from build123d import *

# Parameters (mm, degrees)
SKETCH022_AS_DRAWN_R                      = 2.7
EXTRUDE013_DEPTH                          = 25.4
EXTRUDE013_ONTO_SKETCH022_PLACEMENT_ANGLE = 8
SKETCH018_AS_DRAWN_R                      = 1.2
EXTRUDE009_DEPTH                          = 7.8
EXTRUDE009_ONTO_SKETCH018_PLACEMENT_ANGLE = 8
EXTRUDE012_DEPTH                          = 6.35
EXTRUDE012_ONTO_SKETCH021_PLACEMENT_ANGLE = 8


with BuildPart() as top_led_holes:
    # Sketch022 as drawn → Extrude013 (new, symmetric)
    with BuildSketch(Plane.XY):
        with Locations((116.082414, 49.440535)):
            Circle(SKETCH022_AS_DRAWN_R)
        with Locations((97.448702, 45.479818)):
            Circle(SKETCH022_AS_DRAWN_R)
        with Locations((78.81499, 41.5191)):
            Circle(SKETCH022_AS_DRAWN_R)
    extrude(amount=EXTRUDE013_DEPTH, both=True)


with BuildPart() as top_led_holes_1:
    # Extrude013 onto Sketch022 placement: moved
    add(top_led_holes.part.moved(Location((42.3672, 0, 47.625))).rotate(Axis((42.3672, 0, 47.625), (0, 1, 0)), EXTRUDE013_ONTO_SKETCH022_PLACEMENT_ANGLE))


with BuildPart() as screw_hole_cuts:
    # Sketch018 as drawn → Extrude009 (new)
    with BuildSketch(Plane.XY):
        with Locations((-31.998318, 84.649891)):
            Circle(SKETCH018_AS_DRAWN_R)
        with Locations((-31.998318, -89.695043)):
            Circle(SKETCH018_AS_DRAWN_R)
        with Locations((156.654735, -49.595599)):
            Circle(SKETCH018_AS_DRAWN_R)
        with Locations((156.654735, 84.649891)):
            Circle(SKETCH018_AS_DRAWN_R)
    extrude(amount=EXTRUDE009_DEPTH)


with BuildPart() as screw_hole_cuts_1:
    # Extrude009 onto Sketch018 placement: moved
    add(screw_hole_cuts.part.moved(Location((39.98734, 0, 30.691416))).rotate(Axis((39.98734, 0, 30.691416), (0, 1, 0)), EXTRUDE009_ONTO_SKETCH018_PLACEMENT_ANGLE))


with BuildPart() as cut006:
    # Sketch021 as drawn → Extrude012 (new)
    with BuildSketch(Plane.XY):
        Polygon((-39.826537, 91.531891), (-39.826537, -98.44048), (161.021837, -55.74884), (163.536735, -52.643218), (163.536735, 88.356895), (160.361736, 91.531891), align=None)
    extrude(amount=EXTRUDE012_DEPTH)


with BuildPart() as cut006_1:
    # Extrude012 onto Sketch021 placement: moved
    add(cut006.part.moved(Location((40.182182, 0, 32.077791))).rotate(Axis((40.182182, 0, 32.077791), (0, 1, 0)), EXTRUDE012_ONTO_SKETCH021_PLACEMENT_ANGLE))

    # Cut004: cut Screw Hole Cuts
    add(screw_hole_cuts_1.part, mode=Mode.SUBTRACT)

    # Cut006: cut Top LED Holes
    add(top_led_holes_1.part, mode=Mode.SUBTRACT)


solid = cut006_1.part
Design review of the part built by this model. Coordinates are the model's own, in mm. Round coordinates to 2 decimals unless told otherwise and drop trailing zeros. Write each loop counter-clockwise with the first axis right and the second up, starting at its lowest first coordinate (ties: lowest second). Pieces come first, ordered by that corner, then holes. Notation, with made-up numbers: (19, 83.5) - (25, 83.5) arc R21 cw to (25, 102.5) - close; hole circle Ø11 at (-24, 80). An arc over 180 degrees is marked (long way). Return JSON: item names as keys, results as strings. Group by question number.
Item 1: For probe 1 along Z at (x, y) = (158.5, -37); probe 2 along Z at (x, y) = (118.5, 16.5); probe 3 along Y at (x, z) = (78, 33), list the stretches that pass through material, from the lowest coordinate up. Write a range as [from, to].
Item 2: The part is to be moulded in two halves that separate along Y. For faces 1 (the face through (100.909, -2.124, 29.956)), 2 (the face through (152.912, 49.559, 19.486)), 3 (the face through (102, 91.532, 27)), say which applies: pulls with the +Y half, pulls with the -Y half, needs draft (parallel to the pull), parting line crosses it, or undercut.
Item 3: We need section B-B on x = 25. Write out the cut boundary in (y, z).
Item 4: Insertion check: P1, Ø10, axis at y = -9, z = 33, coming from the -X side; P2, Ø4, axis at x = 127, z = 17.5, coming from the -Y side; P3, Ø8, axis at x = 30, y = 23, coming from the -Z side. Each pin has a flat end and moves straight along its axis. Give the tip position at first contact, or say it passes through.
Item 5: We need section A-A on y = 62.5. Write out the cut boundary in (x, z), and give its area (3 significant figures).
Model answer:
{
 "1": {"probe 1": "z = [15.45, 21.86]", "probe 2": "z = [21.07, 27.48]", "probe 3": "y = [-82.04, 91.53]"},
 "2": {"face 1": "needs draft", "face 2": "undercut", "face 3": "pulls with the +Y half"},
 "3": {"outline": "(-93.42, 40.62) - (-93.23, 34.21) - (91.53, 34.21) - (91.53, 40.62) - close"},
 "4": {"P1": "stops at x = 0.74", "P2": "passes through", "P3": "stops at z = 32.95"},
 "5": {"outline": "(0.74, 37.62) - (202.13, 9.32) - (203.01, 15.61) - (1.63, 43.91) - close", "area": "1,290 mm²"}
}
